Design review of the part built by this model. Coordinates are the model's own, in mm. Round coordinates to 2 decimals unless told otherwise and drop trailing zeros. Loops run counter-clockwise (first coordinate to the right, second up) from the corner with the lowest first, then second, coordinate; pieces in that order, holes last. Notation, with made-up numbers: (33, -15) -> (53, -15) arc R13 ccw to (53, -8) -> close; hole circle Ø1 at (86.25, 77). An arc over 180 degrees is marked (long way). Write each question's results on one line, items separated by ' | '. Start each with the question number.
from build123d import *

# Parameters (mm, degrees)
SKETCH2_W           = 26
SKETCH2_H           = 6
BOSS_EXTRUDE1_DEPTH = 10
SKETCH3_R           = 0.5
CUT_EXTRUDE1_DEPTH  = 5
SKETCH4_W           = 0.5
SKETCH4_H           = 3
BOSS_EXTRUDE2_DEPTH = 0.5


with BuildPart() as part:
    # Sketch2 → Boss-Extrude1 (new body)
    with BuildSketch(Plane.XY):
        with Locations((13, 3)):
            Rectangle(SKETCH2_W, SKETCH2_H)
    extrude(amount=BOSS_EXTRUDE1_DEPTH)

    # Sketch3 → Cut-Extrude1 (cut)
    with BuildSketch(Plane.XY.offset(10)):
        with Locations((1.125, 2)):
            Circle(SKETCH3_R)
        with Locations((2.375, 2)):
            Circle(SKETCH3_R)
        with Locations((3.625, 2)):
            Circle(SKETCH3_R)
        with Locations((4.875, 2)):
            Circle(SKETCH3_R)
        with Locations((6.125, 2)):
            Circle(SKETCH3_R)
        with Locations((7.375, 2)):
            Circle(SKETCH3_R)
        with Locations((8.625, 2)):
            Circle(SKETCH3_R)
        with Locations((9.875, 2)):
            Circle(SKETCH3_R)
        with Locations((11.125, 2)):
            Circle(SKETCH3_R)
        with Locations((12.375, 2)):
            Circle(SKETCH3_R)
        with Locations((13.625, 2)):
            Circle(SKETCH3_R)
        with Locations((14.875, 2)):
            Circle(SKETCH3_R)
        with Locations((16.125, 2)):
            Circle(SKETCH3_R)
        with Locations((17.375, 2)):
            Circle(SKETCH3_R)
        with Locations((18.625, 2)):
            Circle(SKETCH3_R)
        with Locations((19.875, 2)):
            Circle(SKETCH3_R)
        with Locations((21.125, 2)):
            Circle(SKETCH3_R)
        with Locations((22.375, 2)):
            Circle(SKETCH3_R)
        with Locations((23.625, 2)):
            Circle(SKETCH3_R)
        with Locations((24.875, 2)):
            Circle(SKETCH3_R)
    cut_extrude1 = extrude(amount=-CUT_EXTRUDE1_DEPTH, mode=Mode.SUBTRACT)

    # Sketch4 → Boss-Extrude2 (add)
    with BuildSketch(Plane(origin=(0, 0, 0), x_dir=(-1, 0, 0), z_dir=(0, -1, 0))):
        with Locations((-24.65, 1.5)):
            Rectangle(SKETCH4_W, SKETCH4_H)
        with Locations((-25.75, 1.5)):
            Rectangle(SKETCH4_W, SKETCH4_H)
        with Locations((-23.55, 1.5)):
            Rectangle(SKETCH4_W, SKETCH4_H)
        with Locations((-22.45, 1.5)):
            Rectangle(SKETCH4_W, SKETCH4_H)
        with Locations((-21.35, 1.5)):
            Rectangle(SKETCH4_W, SKETCH4_H)
        with Locations((-20.25, 1.5)):
            Rectangle(SKETCH4_W, SKETCH4_H)
        with Locations((-19.15, 1.5)):
            Rectangle(SKETCH4_W, SKETCH4_H)
        with Locations((-18.05, 1.5)):
            Rectangle(SKETCH4_W, SKETCH4_H)
        with Locations((-16.95, 1.5)):
            Rectangle(SKETCH4_W, SKETCH4_H)
        with Locations((-15.85, 1.5)):
            Rectangle(SKETCH4_W, SKETCH4_H)
        with Locations((-14.75, 1.5)):
            Rectangle(SKETCH4_W, SKETCH4_H)
        with Locations((-13.65, 1.5)):
            Rectangle(SKETCH4_W, SKETCH4_H)
        with Locations((-12.55, 1.5)):
            Rectangle(SKETCH4_W, SKETCH4_H)
        with Locations((-11.45, 1.5)):
            Rectangle(SKETCH4_W, SKETCH4_H)
        with Locations((-10.35, 1.5)):
            Rectangle(SKETCH4_W, SKETCH4_H)
        with Locations((-9.25, 1.5)):
            Rectangle(SKETCH4_W, SKETCH4_H)
        with Locations((-8.15, 1.5)):
            Rectangle(SKETCH4_W, SKETCH4_H)
        with Locations((-7.05, 1.5)):
            Rectangle(SKETCH4_W, SKETCH4_H)
        with Locations((-5.95, 1.5)):
            Rectangle(SKETCH4_W, SKETCH4_H)
        with Locations((-4.85, 1.5)):
            Rectangle(SKETCH4_W, SKETCH4_H)
        with Locations((-3.75, 1.5)):
            Rectangle(SKETCH4_W, SKETCH4_H)
        with Locations((-2.65, 1.5)):
            Rectangle(SKETCH4_W, SKETCH4_H)
        with Locations((-1.55, 1.5)):
            Rectangle(SKETCH4_W, SKETCH4_H)
        with Locations((-0.45, 1.5)):
            Rectangle(SKETCH4_W, SKETCH4_H)
    extrude(amount=-BOSS_EXTRUDE2_DEPTH)

    # Mirror1: Cut-Extrude1 across plane
    add(cut_extrude1.mirror(Plane(origin=(0, 3, 0), x_dir=(0, 0, 1), z_dir=(0, -1, 0))), mode=Mode.SUBTRACT)


solid = part.part
1) Take a section at A-A (z = 6.5). State how many separate pieces and enclosed holes the cut face has, plus the area to 3 significant figures.
2) Insertion check: pin 1 (0.5 mm diameter, centred on x = 3.5, y = 4, fed in from +Z); pin 2 (1 mm diameter, centred on x = 13.5, y = 3, fed in from -Z); pin 3 (0.6 mm diameter, centred on x = 16, z = -1.5, fed in from +Y); pin 4 (0.5 mm diameter, centred on x = 14, y = 2, fed in from +Z). Each pin has a flat end and moves straight along its axis. Give the tip position at first contact, or say it passes through.
3) To check wall thickness, follow line 1 (Y direction, x = 16.5, z = 5.25); line 2 (Y direction, x = 3.5, z = 6.75); line 3 (Z direction, x = 2, y = 1.2). State the ranges of each line that lie inside material, in increasing order. Write a range as from..to.
4) The part is to be moulded in two halves that separate along X. For faces 1 (the face through (7.4, 2, 5)), 2 (the face through (7.85, 3.85, 7.54)), say which applies: +X half, -X half, draft (parallel to the pull), parting line (faces both ways), or undercut.
5) Take a section at B-B (y = 2.75). Write out the cut boundary in (x, z).
Geometry check:
1) separate pieces: 1 | enclosed holes: 40 | area: 125 mm^2
2) pin 1: stops at z = 5 | pin 2: stops at z = 0 | pin 3: stops at y = 0.5 | pin 4: stops at z = 10
3) line 1: y = 0..1.67, 2.33..3.67, 4.33..6 | line 2: y = 0..1.52, 2.48..3.52, 4.48..6 | line 3: z = 0..10
4) face 1: undercut | face 2: undercut
5) outline: (0, 0) -> (26, 0) -> (26, 10) -> (0, 10) -> close
